from build123d import *

# Parameters (mm, degrees)
F0_W     = 30
F0_H     = 2.5
F1_DEPTH = 2
F0_H_2   = 7.5
F0_R     = 1.7
F2_DEPTH = 4.75
F0_H_3   = 2
F3_DEPTH = 6.75
F4_R     = 1.99999


# Not quite as in the source:
# - a fillet or chamfer is up to 0.001 mm smaller than in the source, because OpenCascade refuses the exact size


with BuildPart() as f1:
    # F0 (on Top) → F1 (new body)
    with BuildSketch(Plane.XY):
        with Locations((7.8400733322, 0.8872417808)):
            Rectangle(F0_W, F0_H)
    extrude(amount=F1_DEPTH)

    # F0 (on Top) → F2 (join)
    with BuildSketch(Plane.XY):
        with Locations((7.8400733322, -4.1127582192)):
            Rectangle(F0_W, F0_H_2)
        with Locations((7.8400733322, -4.8627582192)):
            Circle(F0_R, mode=Mode.SUBTRACT)
    extrude(amount=F2_DEPTH)

    # F0 (on Top) → F3 (join)
    with BuildSketch(Plane.XY):
        with Locations((7.8400733322, -8.8627582192)):
            Rectangle(F0_W, F0_H_3)
    extrude(amount=F3_DEPTH)

    # F4 (radius 2 in the source; OpenCascade refuses exactly that, so slightly less here)
    f4_edges = [f1.edges().sort_by_distance(p)[0] for p in [
        (-7.159927, 2.137242, 1),
        (22.840073, 2.137242, 1),
        (-7.159927, -9.862758, 3.375),
        (22.840073, -9.862758, 3.375),
        (7.840073, 2.137242, 0),
        (22.840073, -3.862758, 0),
        (-7.159927, -3.862758, 0),
        (7.840073, -9.862758, 0),
        (7.840073, -9.862758, 6.75),
    ]]
    fillet(f4_edges, radius=F4_R)


solid = f1.part
The listing builds one solid part. Answer for the finished solid, in the listing's coordinates (mm). A direction names the side the tool comes from. Round coordinates to 2 decimals unless told otherwise and drop trailing zeros. Order: outer loops, then holes, each group sorted by start corner. A loop starts at its lowest first (then second) coordinate and runs counter-clockwise, first axis right, second up. Notation, with made-up numbers: (-5, -35) -> (9, -35) arc R16 cw to (9, -12) -> close; hole circle Ø6 at (-12.5, 29.25). An arc over 180 degrees is marked (long way). Put each result on its own line as item: value.
Q1. Which of the six approach directions +Z, -Z, +X, -X, +Y, -Y give full straight-line access (tool end or side, diameter ignored) to faces 1 (the flat face through (8, 1, 2)), 2 (the cylindrical face through (8.05, -9.26, 6.18))?
Results list:
face 1: +Z, +X, -X, +Y
face 2: +Z, +X, -X, -Y
Q2. Section B-B, the plane z = 3.5 is taken. Write down the section's boundary in (x, y), and give its area (3 significant figures).
Results list:
outline: (-7.16, -7.86) arc R2 ccw to (-5.16, -9.86) -> (20.84, -9.86) arc R2 ccw to (22.84, -7.86) -> (22.84, -0.36) -> (-7.16, -0.36) -> close; hole circle Ø3.4 at (7.84, -4.86)
area: 274 mm^2
Q3. Section D-D, the plane y = -3.5 is taken. Write down the section's boundary in (x, z).
Results list:
outline: (-7.16, 2) arc R2 ccw to (-5.16, 0) -> (6.82, 0) -> (6.82, 4.75) -> (-7.16, 4.75) -> close; (8.86, 0) -> (20.84, 0) arc R2 ccw to (22.84, 2) -> (22.84, 4.75) -> (8.86, 4.75) -> close
Q4. Consider line 1 along Y through (x, z) = (10, 3); line 2 along Z through (x, y) = (3, 0); line 3 along Z through (x, y) = (-4.25, -4.75). Determine where each line is inside the solid, lowest interval first.
Results list:
line 1: -9.86 to -0.36
line 2: 0 to 2
line 3: 0 to 4.75
Q5. Each of these flat-tipped pins is pushed along its axis until it touches: P1, Ø2, axis at x = -3.5, z = 3.5, coming from the +Y side; P2, Ø1.5, axis at x = 4, z = 1, coming from the -Y side; P3, Ø0.6, axis at x = 6.5, z = 5.5, coming from the +Y side; P4, Ø2.5, axis at x = 7.84, y = -4.86, coming from the +Z side. Where does it stop, or does it pass through?
Results list:
P1: y = -0.36
P2: y = -9.85
P3: y = -7.86
P4: through
